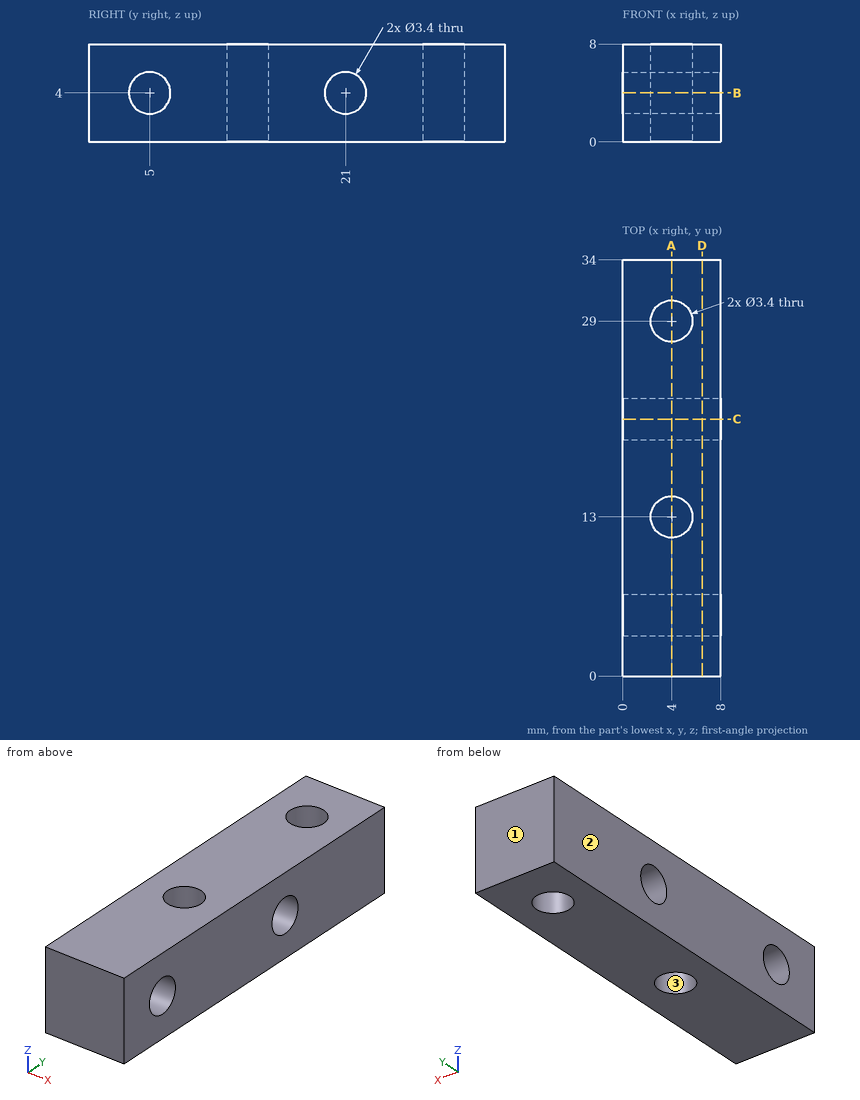
Here's the drawing with two shaded views (mm, measured from the low corner). I have some questions. Coordinates: 2 decimals unless noted, no trailing zeros. Order: outer loops, then holes, each group sorted by start corner. A loop starts at its lowest first (then second) coordinate and runs counter-clockwise, first axis right, second up. Notation, with made-up numbers: (-19.5, 32.25) - (20.5, 32.25) arc R13 cw to (20.5, 56.25) - close; hole circle Ø4 at (2, -22). An arc over 180 degrees is marked (long way). Answer in a Markdown table with one row per item. Add a question column.
(1) If we section it at C-C, the plane y = 21: Please give me the cut outline in (x, z), then the cut area to 3 significant figures.
(2) I need wall thicknesses on L1, parallel to Y at x = 2, z = 4; L2, parallel to Y at x = 4.25, z = 7.25; L3, parallel to Y at x = 4, z = 5.5. Which ranges of each line are inside material? Lowest first, please.
(3) If we mould it in two halves opening along Y, with no side actions, what happens to the marked faces 1, 2 and 3? For each: released by +Y, released by -Y, zero draft, split by the parting line, or undercut.
(4) If we section it at D-D, the plane x = 6.5: Please give me the cut outline in (y, z), then the cut area to 3 significant figures.
(5) If we section it at A-A, the plane x = 4: Please give me the cut outline in (y, z), then the cut area to 3 significant figures.
(6) Will these pins go through, and if not, where does the flat tip stop? pin 1 (2 mm diameter, centred on x = 4, y = 29, fed in from -Z); pin 2 (4 mm diameter, centred on y = 23, z = 1, fed in from -X).
(7) If we section it at B-B, the plane z = 4: Please give me the cut outline in (x, y), then the cut area to 3 significant figures.
Results are:
| question | item | result |
|---|---|---|
| 1 | outline | (0, 0) - (8, 0) - (8, 2.3) - (0, 2.3) - close; (0, 5.7) - (8, 5.7) - (8, 8) - (0, 8) - close |
| 1 | area | 36.8 mm2 |
| 2 | L1 | y = 0 to 3.3, 6.7 to 19.3, 22.7 to 34 |
| 2 | L2 | y = 0 to 11.32, 14.68 to 27.32, 30.68 to 34 |
| 2 | L3 | y = 0 to 4.2, 5.8 to 11.3, 14.7 to 20.2, 21.8 to 27.3, 30.7 to 34 |
| 3 | face 1 | released by +Y |
| 3 | face 2 | zero draft |
| 3 | face 3 | undercut |
| 4 | outline | (0, 0) - (34, 0) - (34, 8) - (0, 8) - close; hole circle Ø3.4 at (5, 4); hole circle Ø3.4 at (21, 4) |
| 4 | area | 254 mm2 |
| 5 | outline | (0, 0) - (11.3, 0) - (11.3, 8) - (0, 8) - close; (14.7, 0) - (27.3, 0) - (27.3, 8) - (14.7, 8) - close; (30.7, 0) - (34, 0) - (34, 8) - (30.7, 8) - close; hole circle Ø3.4 at (5, 4); hole circle Ø3.4 at (21, 4) |
| 5 | area | 199 mm2 |
| 6 | pin 1 | passes through |
| 6 | pin 2 | stops at x = 0 |
| 7 | outline | (0, 0) - (8, 0) - (8, 3.3) - (0, 3.3) - close; (0, 6.7) - (8, 6.7) - (8, 19.3) - (0, 19.3) - close; (0, 22.7) - (8, 22.7) - (8, 34) - (0, 34) - close; hole circle Ø3.4 at (4, 13); hole circle Ø3.4 at (4, 29) |
| 7 | area | 199 mm2 |
